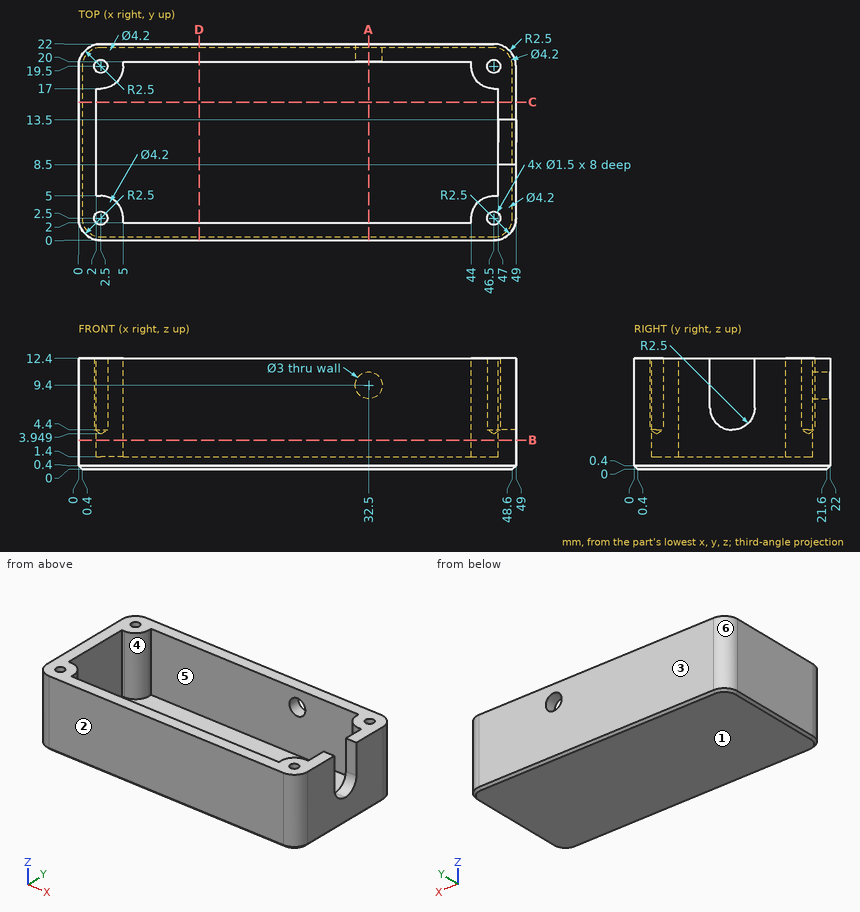
Geometry: see drawing. Coordinates: mm, zero at the bounding-box minimum. A direction names the side the tool comes from. Coordinates: 2 decimals unless noted, no trailing zeros. Loops run counter-clockwise (first coordinate to the right, second up) from the corner with the lowest first, then second, coordinate; pieces in that order, holes last. Notation, with made-up numbers: M 80.5,27 L 134.5,27 A22 ccw 134.5,58 Z; hole C 67.5,-28 d2. An arc over 180 degrees is marked long. Put each result on its own line as item: value. Start each with the question number.
1) Cut plane B-B on z = 3.25. Return the cut outline in (x, y), then the cut area to 3 significant figures.
2) Cut plane D-D on x = 13.5. Return the cut outline in (y, z).
3) Ray query, L1, parallel to Y at x = 46.5, z = 8.5; L2, parallel to X at y = 19.5, z = 11; L3, parallel to Y at x = 14, z = 10. Return the intervals inside material, ascending. Write a range as from..to.
4) Cut plane A-A on x = 32.5. Return the cut outline in (y, z).
5) Cut plane C-C on y = 15.5. Return the cut outline in (x, z).
6) Pull-direction query (Y, two-part tool) for the marked faces 1, 2, 3 and 4; classes: pulls with the +Y half, pulls with the -Y half, needs draft (parallel to the pull), parting line crosses it, or undercut.
7) Reachability of the marked faces 5 and 6 from +Z, -Z, +X, -X, +Y, -Y: full face, straight path, thin tool, end or side. Return the list, or none.
8) Contact query for flat-ended pins moving along their axis: pin 1 Ø1.6 at (x, z) = (47.5, 11) entering from +Y; pin 2 Ø0.6 at (x, z) = (2, 6.5) entering from -Y; pin 3 Ø9 at (x, y) = (26.5, 8) entering from +Z. Output: stop coordinate, or through.
The answers:
1. outline: M 0,2.5 A2.5 ccw 2.5,0 L 46.5,0 A2.5 ccw 49,2.5 L 49,19.5 A2.5 ccw 46.5,22 L 2.5,22 A2.5 ccw 0,19.5 Z; hole M 2,5 L 2.5,5 A2.5 cw 5,2.5 L 5,2 L 44,2 L 44,2.5 A2.5 cw 46.5,5 L 47,5 L 47,17 L 46.5,17 A2.5 cw 44,19.5 L 44,20 L 5,20 L 5,19.5 A2.5 cw 2.5,17 L 2,17 Z
1. area: 293 mm²
2. outline: M 0,0.4 L 0.4,0 L 21.6,0 L 22,0.4 L 22,12.4 L 20,12.4 L 20,1.4 L 2,1.4 L 2,12.4 L 0,12.4 Z
3. L1: y = 0..1.75, 3.25..5, 17..18.75, 20.25..22
3. L2: x = 0..1.75, 3.25..5, 44..45.75, 47.25..49
3. L3: y = 0..2, 20..22
4. outline: M 0,0.4 L 0.4,0 L 21.6,0 L 22,0.4 L 22,7.9 L 20,7.9 L 20,1.4 L 2,1.4 L 2,12.4 L 0,12.4 Z; M 20,10.9 L 22,10.9 L 22,12.4 L 20,12.4 Z
5. outline: M 0,0.4 L 0.4,0 L 48.6,0 L 49,0.4 L 49,12.4 L 47,12.4 L 47,1.4 L 2,1.4 L 2,12.4 L 0,12.4 Z
6. face 1: needs draft
6. face 2: pulls with the -Y half
6. face 3: pulls with the +Y half
6. face 4: undercut
7. face 5: +Z
7. face 6: +Z, -Z, -X, +Y
8. pin 1: stops at y = 21.99
8. pin 2: stops at y = 0.01
8. pin 3: stops at z = 1.4
